Print and shaded views of the part. All mm, measured from the part's lowest x, y and z. Round coordinates to 2 decimals unless told otherwise and drop trailing zeros. Loops run counter-clockwise (first coordinate to the right, second up) from the corner with the lowest first, then second, coordinate; pieces in that order, holes last. Notation, with made-up numbers: (38.5, 55) - (93.5, 55) arc R30 cw to (93.5, 78) - close; hole circle Ø6 at (64, -14). An arc over 180 degrees is marked (long way). Use one line per item in the form item = value.
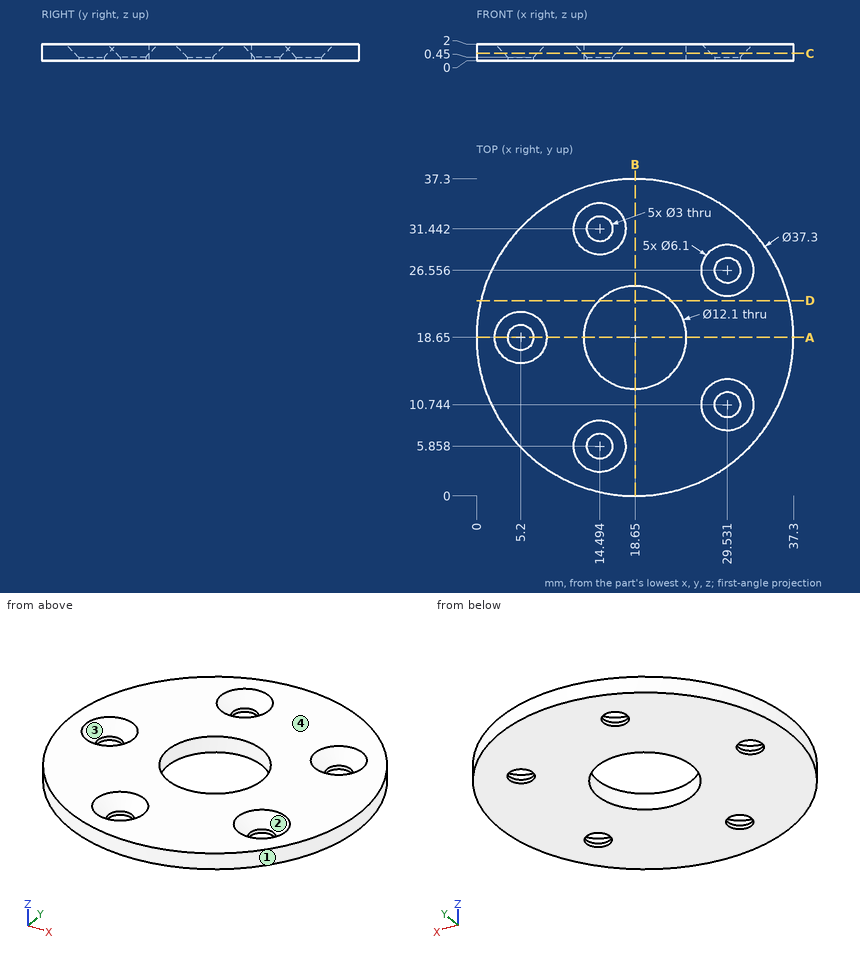
1. Pull direction X, two halves, no side cores. Call the marked faces 1, 2, 3 and 4: +X half, -X half, draft (parallel to the pull), parting line (faces both ways), or undercut.
Geometry check:
face_1 = parting line
face_2 = undercut
face_3 = undercut
face_4 = draft
2. Wall check: probe 1 along Y at (x, z) = (18.65, 0.8); probe 2 along Y at (x, z) = (28.5, 1.9) (1 decimal); probe 3 along X at (y, z) = (18, 0.85) (1 decimal). Give the ranges that are in metal, low to high.
Geometry check:
probe_1 = 0 to 12.6, 24.7 to 37.3
probe_2 = 2.8 to 8, 13.5 to 23.8, 29.3 to 34.5
probe_3 = 0 to 3.4, 7 to 12.6, 24.7 to 37.3
3. Cut at A-A, the plane y = 18.65. Give the cut face in (x, z), plus the area to 3 significant figures.
Geometry check:
outline = (0, 0) - (3.7, 0) - (3.7, 0.45) - (2.15, 2) - (0, 2) - close; (6.7, 0) - (12.6, 0) - (12.6, 2) - (8.25, 2) - (6.7, 0.45) - close; (24.7, 0) - (37.3, 0) - (37.3, 2) - (24.7, 2) - close
area = 42.0 mm^2
4. Cut at D-D, the plane y = 23. Give the cut face in (x, z) (1 decimal).
Geometry check:
outline = (0.5, 0) - (14.4, 0) - (14.4, 2) - (0.5, 2) - close; (22.9, 0) - (36.8, 0) - (36.8, 2) - (22.9, 2) - close
5. Flat gauge pins, fed straight in: pin 1 (2.5 mm diameter, centred on x = 29.53, y = 10.74, fed in from -Z); pin 2 (4 mm diameter, centred on x = 14.49, y = 5.86, fed in from +Z) (1 decimal). Where does each tip first touch, or does it go through?
Geometry check:
pin_1 = through
pin_2 = 1
6. Cut at C-C, the plane z = 0.9. Give the number of separate pieces and of enclosed holes in the cut face, plus the area to 3 significant figures.
Geometry check:
separate_pieces = 1
enclosed_holes = 6
area = 918 mm^2
7. Cut at B-B, the plane x = 18.65. Give the cut face in (y, z), plus the area to 3 significant figures.
Geometry check:
outline = (0, 0) - (12.6, 0) - (12.6, 2) - (0, 2) - close; (24.7, 0) - (37.3, 0) - (37.3, 2) - (24.7, 2) - close
area = 50.4 mm^2
